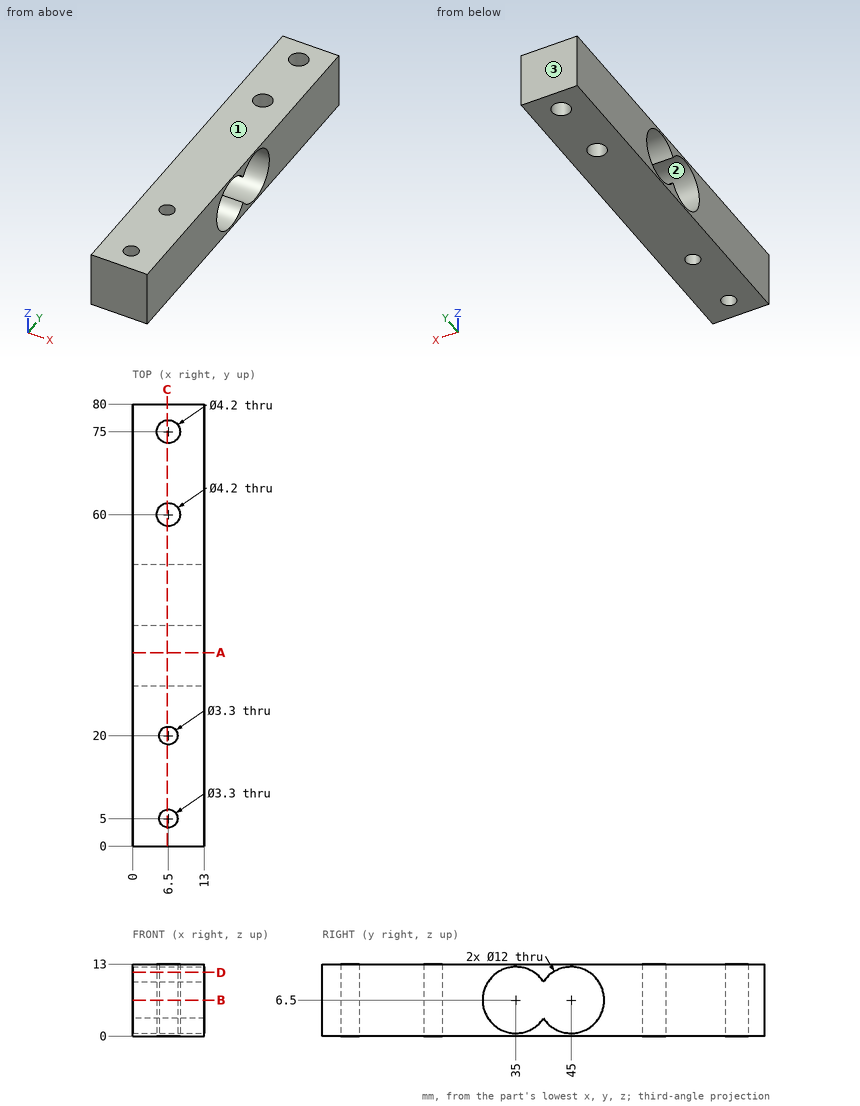
Can you work these out from the drawing? Everything is in mm from the part's minimum corner. Give positions to 0.01 mm unless a question says otherwise; leave off trailing zeros. Order: outer loops, then holes, each group sorted by start corner. A loop starts at its lowest first (then second) coordinate and runs counter-clockwise, first axis right, second up. Notation, with made-up numbers: M -11.5,-17 L 44.5,-17 A27 ccw 44.5,7 Z; hole C -36.5,1.25 d2. An arc over 180 degrees is marked long. Use a Markdown table: item, result. Add a question column.
Item 1: Suppose I cut it at D-D (z = 11.5). List the corners of the cut face in (x, y) for me.
Item 2: Suppose I cut it at B-B (z = 6.5). List the corners of the cut face in (x, y) for me.
Item 3: Suppose I cut it at A-A (y = 35). List the corners of the cut face in (x, z) for me, then the cut area to 3 significant figures.
Item 4: We'd pull the mould along Z, two halves only. Please class the marked faces 1, 2 and 3: +Z half, -Z half, draft (parallel to the pull), parting line (faces both ways), or undercut.
Item 5: If I drill on L1, parallel to Y at x = 6.5, z = 6.25; L2, parallel to Y at x = 6.5, z = 3.5; L3, parallel to Y at x = 1.5, z = 10.25, over which ranges is the centre line in solid material (lowest first)? Write a range as [from, to].
Item 6: Suppose I cut it at C-C (x = 6.25). List the corners of the cut face in (y, z) for me, then the cut area to 3 significant figures.
Answer sheet:
| question | item | result |
|---|---|---|
| 1 | outline | M 0,0 L 13,0 L 13,31.68 L 0,31.68 Z; M 0,38.32 L 13,38.32 L 13,41.68 L 0,41.68 Z; M 0,48.32 L 13,48.32 L 13,80 L 0,80 Z; hole C 6.5,60 d4.2; hole C 6.5,75 d4.2; hole C 6.5,5 d3.3; hole C 6.5,20 d3.3 |
| 2 | outline | M 0,0 L 13,0 L 13,29 L 0,29 Z; M 0,51 L 13,51 L 13,80 L 0,80 Z; hole C 6.5,60 d4.2; hole C 6.5,75 d4.2; hole C 6.5,5 d3.3; hole C 6.5,20 d3.3 |
| 3 | outline | M 0,0 L 13,0 L 13,0.5 L 0,0.5 Z; M 0,12.5 L 13,12.5 L 13,13 L 0,13 Z |
| 3 | area | 13.0 mm² |
| 4 | face 1 | +Z half |
| 4 | face 2 | undercut |
| 4 | face 3 | draft |
| 5 | L1 | y = [0, 3.35], [6.65, 18.35], [21.65, 29.01], [50.99, 57.9], [62.1, 72.9], [77.1, 80] |
| 5 | L2 | y = [0, 3.35], [6.65, 18.35], [21.65, 29.8], [50.2, 57.9], [62.1, 72.9], [77.1, 80] |
| 5 | L3 | y = [0, 30.32], [39.68, 40.32], [49.68, 80] |
| 6 | outline | M 0,0 L 3.37,0 L 3.37,13 L 0,13 Z; M 6.63,0 L 18.37,0 L 18.37,13 L 6.63,13 Z; M 21.63,0 L 57.91,0 L 57.91,13 L 21.63,13 Z; M 62.09,0 L 72.91,0 L 72.91,13 L 62.09,13 Z; M 77.09,0 L 80,0 L 80,13 L 77.09,13 Z; hole M 40,3.18 A6 ccw long 40,9.82 A6 ccw long Z |
| 6 | area | 630 mm² |
